Part model, mm, in its own coordinate system. A direction names the side the tool comes from. Round coordinates to 2 decimals unless told otherwise and drop trailing zeros. Write each loop counter-clockwise with the first axis right and the second up, starting at its lowest first coordinate (ties: lowest second). Pieces come first, ordered by that corner, then holes.
from build123d import *

# Parameters (mm, degrees)
F1_DEPTH = 3
F2_R     = 86.474074


with BuildPart() as f1:
    # F0 (on Front) → F1 (new body)
    with BuildSketch(Plane.XZ):
        with BuildLine():
            Line((38.813758, -39.944117), (14.887724, -1.831849))
            ThreePointArc((14.887724, -1.831849), (11.719036, 9.362916), (1.5, 14.924812))
            Line((1.5, 14.924812), (1.5, 9.863055))
            Line((1.5, 9.863055), (-1.5, 9.863055))
            Line((-1.5, 9.863055), (-1.5, 14.924812))
            ThreePointArc((-1.5, 14.924812), (-11.719036, 9.362916), (-14.887724, -1.831849))
            Line((-14.887724, -1.831849), (-38.813758, -39.944117))
            Line((-38.813758, -39.944117), (-22.813758, -39.944117))
            Line((-22.813758, -39.944117), (0, 0))
            Line((0, 0), (22.813758, -39.944117))
            Line((22.813758, -39.944117), (38.813758, -39.944117))
        make_face()
    extrude(amount=F1_DEPTH)

    # F2
    f2_edges = [f1.edges().sort_by_distance(p)[0] for p in [
        (14.887724, -1.5, -1.831849),
        (-14.887724, -1.5, -1.831849),
    ]]
    fillet(f2_edges, radius=F2_R)


solid = f1.part
Q1. Tool access for faces 1 (the cylindrical face through (9.58, -1.48, 11.54)), 2 (the flat face through (11.247, -1.479, -19.692)), 3 (the flat face through (0, -1, 9.863)): list every direction of +Z, -Z, +X, -X, +Y, -Y with a clear straight run to the whole face (end or side of a thin tool).
Q2. Drop flat-ended pins along their axis: P1, Ø8, axis at x = 28.5, z = -10.5, coming from the -Y side; P2, Ø1.5, axis at x = 0, y = -1.5, coming from the +Z side; P3, Ø0.9, axis at y = -2, z = 12.5, coming from the -X side. Give the stop position or say it passes through.
Q3. Saw through at B-B, the plane y = -1.25. Write the cut outline in (x, z), and give its area (3 significant figures).
Q4. Saw through at A-A, the plane z = -33.5. Write the cut outline in (x, y), and give its area (3 significant figures).
Q5. Saw through at D-D, the plane x = -25. Write the cut outline in (y, z), and give its area (3 significant figures).
Q6. Wall check: line 1 (X direction, y = -0.05, z = -36); line 2 (X direction, y = -0.9, z = -37); line 3 (Z direction, x = -25, y = -2.45). Give the ranges that are in metal, low to high.
Q7. Saw through at C-C, the plane z = -14. Write the cut outline in (x, y), and give its area (3 significant figures).
Computed:
1. face 1: +Z, +X, +Y, -Y
1. face 2: -Z, +Y, -Y
1. face 3: +Z, +Y, -Y
2. P1: passes through
2. P2: stops at z = 9.86
2. P3: stops at x = -8.93
3. outline: (-38.81, -39.94) - (-22.81, -39.94) - (0, 0) - (22.81, -39.94) - (38.81, -39.94) - (23.63, -15.76) arc R86.47 cw to (14.32, 4.47) arc R15 ccw to (1.5, 14.92) - (1.5, 9.86) - (-1.5, 9.86) - (-1.5, 14.92) arc R15 ccw to (-14.32, 4.47) arc R86.47 cw to (-23.63, -15.76) - close
3. area: 1,550 mm2
4. outline: (-34.77, -3) - (-19.13, -3) - (-19.13, 0) - (-34.77, 0) - close; (19.13, -3) - (34.77, -3) - (34.77, 0) - (19.13, 0) - close
4. area: 93.8 mm2
5. outline: (-3, -39.94) - (0, -39.94) - (0, -17.94) - (-3, -17.94) - close
5. area: 66.0 mm2
6. line 1: x = -36.34 to -20.56, 20.56 to 36.34
6. line 2: x = -36.97 to -21.13, 21.13 to 36.97
6. line 3: z = -39.94 to -17.94
7. outline: (-22.56, -3) - (-8, -3) - (-8, 0) - (-22.56, 0) - close; (8, -3) - (22.56, -3) - (22.56, 0) - (8, 0) - close
7. area: 87.4 mm2
